```python
from build123d import *

# Parameters (mm, degrees)
CROQUIS1_W              = 3
CROQUIS1_H              = 20
CROQUIS1_W_2            = 300
CROQUIS1_H_2            = 60
SALIENTE_EXTRUIR1_DEPTH = 3


with BuildPart() as part:
    # Croquis1 → Saliente-Extruir1 (new body)
    with BuildSketch(Plane(origin=(0, 0, 0), x_dir=(1, 0, 0), z_dir=(0, 1, 0))):
        Polygon((155, -80), (162, -80), (165, -80), (165, -77), (162, -77), (162, -65.002891293), (165, -65.002891293), (165, 64.997108707), (162, 64.997108707), (162, 77), (165, 77), (165, 80), (162, 80), (155, 80), (155, 77), (145, 77), (145, 80), (135, 80), (135, 77), (125, 77), (125, 80), (115, 80), (115, 77), (105, 77), (105, 80), (95, 80), (95, 77), (85, 77), (85, 80), (75, 80), (75, 77), (65, 77), (65, 80), (55, 80), (55, 77), (45, 77), (45, 80), (35, 80), (35, 77), (25, 77), (25, 80), (15, 80), (15, 77), (5, 77), (5, 80), (-5, 80), (-5, 77), (-15, 77), (-15, 80), (-25, 80), (-25, 77), (-35, 77), (-35, 80), (-45, 80), (-45, 77), (-55, 77), (-55, 80), (-65, 80), (-65, 77), (-75, 77), (-75, 80), (-85, 80), (-85, 77), (-95, 77), (-95, 80), (-105, 80), (-105, 77), (-115, 77), (-115, 80), (-125, 80), (-125, 77), (-135, 77), (-135, 80), (-145, 80), (-145, 77), (-155, 77), (-155, 80), (-165, 80), (-165, 77), (-175, 77), (-175, 80), (-182, 80), (-185, 80), (-185, 77), (-182, 77), (-182, 64.997108707), (-185, 64.997108707), (-185, -65.002891293), (-182, -65.002891293), (-182, -77), (-185, -77), (-185, -80), (-182, -80), (-175, -80), (-175, -77), (-165, -77), (-165, -80), (-155, -80), (-155, -77), (-145, -77), (-145, -80), (-135, -80), (-135, -77), (-125, -77), (-125, -80), (-115, -80), (-115, -77), (-105, -77), (-105, -80), (-95, -80), (-95, -77), (-85, -77), (-85, -80), (-75, -80), (-75, -77), (-65, -77), (-65, -80), (-55, -80), (-55, -77), (-45, -77), (-45, -80), (-35, -80), (-35, -77), (-25, -77), (-25, -80), (-15, -80), (-15, -77), (-5, -77), (-5, -80), (5, -80), (5, -77), (15, -77), (15, -80), (25, -80), (25, -77), (35, -77), (35, -80), (45, -80), (45, -77), (55, -77), (55, -80), (65, -80), (65, -77), (75, -77), (75, -80), (85, -80), (85, -77), (95, -77), (95, -80), (105, -80), (105, -77), (115, -77), (115, -80), (125, -80), (125, -77), (135, -77), (135, -80), (145, -80), (145, -77), (155, -77), align=None)
        with Locations((-165, -30.002891293)):
            Rectangle(CROQUIS1_W, CROQUIS1_H, mode=Mode.SUBTRACT)
        with Locations((-10, 0)):
            Rectangle(CROQUIS1_W_2, CROQUIS1_H_2, mode=Mode.SUBTRACT)
        with Locations((156, -30.002891293)):
            Rectangle(CROQUIS1_W, CROQUIS1_H, mode=Mode.SUBTRACT)
        with Locations((-165, 49.997108707)):
            Rectangle(CROQUIS1_W, CROQUIS1_H, mode=Mode.SUBTRACT)
        with Locations((-165, 9.997108707)):
            Rectangle(CROQUIS1_W, CROQUIS1_H, mode=Mode.SUBTRACT)
        with Locations((145, 9.997108707)):
            Rectangle(CROQUIS1_W, CROQUIS1_H, mode=Mode.SUBTRACT)
        with Locations((145, -30.002891293)):
            Rectangle(CROQUIS1_W, CROQUIS1_H, mode=Mode.SUBTRACT)
        with Locations((145, 49.997108707)):
            Rectangle(CROQUIS1_W, CROQUIS1_H, mode=Mode.SUBTRACT)
        with Locations((156, 49.997108707)):
            Rectangle(CROQUIS1_W, CROQUIS1_H, mode=Mode.SUBTRACT)
        with Locations((156, 9.997108707)):
            Rectangle(CROQUIS1_W, CROQUIS1_H, mode=Mode.SUBTRACT)
    extrude(amount=SALIENTE_EXTRUIR1_DEPTH)


solid = part.part
```
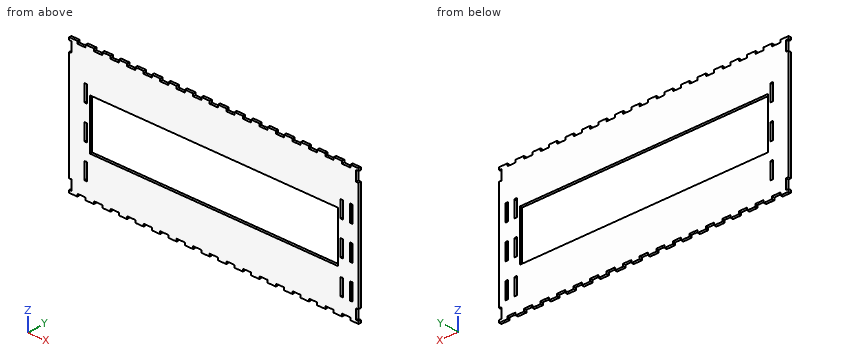
Verification items for the finished model (mm, model axes). Coordinates: 2 decimals unless noted, no trailing zeros. Order: outer loops, then holes, each group sorted by start corner. A loop starts at its lowest first (then second) coordinate and runs counter-clockwise, first axis right, second up. Notation, with made-up numbers: (-22.5, 34.5) - (17.5, 34.5) arc R24 cw to (17.5, 58.5) - close; hole circle Ø8 at (78.25, 30.5). An arc over 180 degrees is marked (long way). Return JSON: item names as keys, results as strings.
(1) Section check C-C, the plane z = -44. Record the cut outline in (x, y).
Filled sheet:
{"outline": "(-185, 0) - (-166.5, 0) - (-166.5, 3) - (-185, 3) - close; (-163.5, 0) - (143.5, 0) - (143.5, 3) - (-163.5, 3) - close; (146.5, 0) - (154.5, 0) - (154.5, 3) - (146.5, 3) - close; (157.5, 0) - (165, 0) - (165, 3) - (157.5, 3) - close"}
(2) Go/stop test with flat-tipped pins: pin 1 (1 mm diameter, centred on x = 54, y = 1.5, fed in from +Z); pin 2 (0.9 mm diameter, centred on x = 72.5, y = 1, fed in from -Z). Record where each tip stops, or that it passes through.
Filled sheet:
{"pin 1": "stops at z = 77", "pin 2": "stops at z = -77"}
(3) Section check A-A, the plane z = 10. Record the cut outline in (x, y), and give its area (3 significant figures).
Filled sheet:
{"outline": "(-185, 0) - (-160, 0) - (-160, 3) - (-185, 3) - close; (140, 0) - (165, 0) - (165, 3) - (140, 3) - close", "area": "150 mm^2"}
(4) Section check D-D, the plane y = 0.6. Give the number of separate pieces and of enclosed holes in the cut face, and give its area (3 significant figures).
Filled sheet:
{"separate pieces": "1", "enclosed holes": "10", "area": "36,300 mm^2"}
(5) Thickness scan on line 1 along X through (y, z) = (1.55, 36.5); line 2 along X through (y, z) = (0.45, -15.5); line 3 along Z through (x, y) = (-20, 0.85). Record the ranges inside material, lowest first.
Filled sheet:
{"line 1": "x = -185 to -166.5, -163.5 to 143.5, 146.5 to 154.5, 157.5 to 165", "line 2": "x = -185 to -166.5, -163.5 to -160, 140 to 143.5, 146.5 to 154.5, 157.5 to 165", "line 3": "z = -80 to -30, 30 to 80"}
(6) Section check B-B, the plane x = -129.5. Record the cut outline in (y, z), and give its area (3 significant figures).
Filled sheet:
{"outline": "(0, -77) - (3, -77) - (3, -30) - (0, -30) - close; (0, 30) - (3, 30) - (3, 77) - (0, 77) - close", "area": "282 mm^2"}
